```python
from build123d import *

# Parameters (mm, degrees)
F0_W            = 37
F0_H            = 21.6
F4_DEPTH        = 50
F5_T            = -2.9
F6_W            = 18.6
F6_H            = 2.5
F7_DEPTH        = 2.9
F8_W            = 36.999993
F8_H            = 21.599919
F9_DEPTH        = 1
F10_D           = 15.5
F10_CBORE_D     = 19
F10_CBORE_DEPTH = 1


with BuildPart() as f4:
    # F0 (on Top) → F4 (new body)
    with BuildSketch(Plane.XY):
        Rectangle(F0_W, F0_H)
    extrude(amount=F4_DEPTH)

    # F5
    f5_openings = [f4.faces().sort_by_distance(p)[0] for p in [
        (0, 0, 50),
        (0, 0, 0),
    ]]
    offset(amount=F5_T, openings=f5_openings)

    # F6 (on face) → F7 (cut)
    with BuildSketch(Plane.YZ.offset(18.5)):
        with Locations((0, 47.25)):
            Rectangle(F6_W, F6_H)
    extrude(amount=-F7_DEPTH, mode=Mode.SUBTRACT)

    # F8 (on offset) → F9 (join)
    with BuildSketch(Plane.XY.offset(50)):
        with Locations((1.5e-05, -3.1e-05)):
            Rectangle(F8_W, F8_H)
    extrude(amount=-F9_DEPTH)

    # F10 (through all)
    with Locations(Plane.XY.offset(50)):
        with Locations((0, 0)):
            CounterBoreHole(F10_D / 2, F10_CBORE_D / 2, F10_CBORE_DEPTH)


solid = f4.part
```
Part model, mm, in its own coordinate system. A direction names the side the tool comes from. Coordinates: 2 decimals unless noted, no trailing zeros. Write each loop counter-clockwise with the first axis right and the second up, starting at its lowest first coordinate (ties: lowest second). Pieces come first, ordered by that corner, then holes.
Item 1: Probe line 1 (Y direction, x = 0, z = 49.55); line 2 (Y direction, x = 6.5, z = 19); line 3 (X direction, y = -6.5, z = 43). List the from-to ranges inside material, lowest first.
Item 2: Pin check, flat tips, straight feed: pin 1 (3 mm diameter, centred on x = 13, y = -0.5, fed in from -Z); pin 2 (1.1 mm diameter, centred on y = 8.5, z = 47.5, fed in from +X). Stop position of each tip, or through.
Item 3: Slice it at D-D (x = 10.5). Write the cut outline in (y, z).
Item 4: Slice it at C-C (z = 13). Write the cut outline in (x, y), and give its area (3 significant figures).
Item 5: Which spindle directions (+Z, -Z, +X, -X, +Y, -Y) get a long thin tool onto all of the face, cutting with end or side? Do faces 4 (the face through (0, -7.9, 24)), 5 (the face through (-18.5, 0, 25)), 6 (the face through (4.38, -8.43, 49.51)), 7 (the face through (18.5, 0, 25)), 8 (the face through (17, 0, 46)). Say none if no direction does.
Item 6: Slice it at B-B (x = 0). Write the cut outline in (y, z).
Item 7: Slice it at A-A (y = 0). Count the separate pieces of the cut face and the enclosed holes in it, and give its area (3 significant figures).
Item 8: Mould opens along Y. For faces 1 (the face through (0, 10.8, 25)), 2 (the face through (18.5, -0.2, 49.5)), 3 (the face through (0, 9, 49)) say: released by +Y, released by -Y, zero draft, split by the parting line, or undercut.
Results found:
1. line 1: y = -10.8 to -9.5, 9.5 to 10.8
1. line 2: y = -10.8 to -7.9, 7.9 to 10.8
1. line 3: x = -18.5 to -15.6, 15.6 to 18.5
2. pin 1: stops at z = 49
2. pin 2: stops at x = 15.6
3. outline: (-10.8, 0) - (-7.9, 0) - (-7.9, 49) - (7.9, 49) - (7.9, 0) - (10.8, 0) - (10.8, 50) - (-10.8, 50) - close
4. outline: (-18.5, -10.8) - (18.5, -10.8) - (18.5, 10.8) - (-18.5, 10.8) - close; hole (-15.6, -7.9) - (15.6, -7.9) - (15.6, 7.9) - (-15.6, 7.9) - close
4. area: 306 mm2
5. face 4: -Z
5. face 5: +Z, -Z, -X, +Y, -Y
5. face 6: +Z
5. face 7: +Z, -Z, +X, +Y, -Y
5. face 8: +X
6. outline: (-10.8, 0) - (-7.9, 0) - (-7.9, 49) - (-9.5, 49) - (-9.5, 50) - (-10.8, 50) - close; (7.9, 0) - (10.8, 0) - (10.8, 50) - (9.5, 50) - (9.5, 49) - (7.9, 49) - close
7. separate pieces: 3
7. enclosed holes: 0
7. area: 295 mm2
8. face 1: released by +Y
8. face 2: zero draft
8. face 3: undercut
